from build123d import *

# Parameters (mm, degrees)
SKETCH_1_W          = 160
SKETCH_1_H          = 140
EXTRUDE_1_DEPTH     = 45
SKETCH_2_W          = 160
SKETCH_2_H          = 100
EXTRUDE_2_DEPTH     = 45
SKETCH_3_R          = 12.5
CUT_EXTRUDE_1_DEPTH = 116.433963806
SKETCH_4_R          = 32.5
CUT_EXTRUDE_2_DEPTH = 157.524758425
SKETCH_5_R          = 50
CUT_EXTRUDE_3_DEPTH = 7.5
SKETCH_7_W          = 136
SKETCH_7_H          = 76
CUT_EXTRUDE_4_DEPTH = 25


with BuildPart() as part:
    # Эскиз1 → Бобышка-Вытянуть1 (new body)
    with BuildSketch(Plane.XY):
        Rectangle(SKETCH_1_W, SKETCH_1_H)
    extrude(amount=EXTRUDE_1_DEPTH)

    # Эскиз2 → Бобышка-Вытянуть2 (add)
    with BuildSketch(Plane.XY.offset(45)):
        with Locations((0, 20)):
            Rectangle(SKETCH_2_W, SKETCH_2_H)
    extrude(amount=EXTRUDE_2_DEPTH)

    # Эскиз3 → Вырез-Вытянуть1 (cut, through all)
    with BuildSketch(Plane.XY.offset(45)):
        with Locations((0, -50)):
            Circle(SKETCH_3_R)
    extrude(amount=-CUT_EXTRUDE_1_DEPTH, mode=Mode.SUBTRACT)

    # Эскиз4 → Вырез-Вытянуть2 (cut, through all)
    with BuildSketch(Plane.XZ.offset(30)):
        with Locations((0, 90)):
            Circle(SKETCH_4_R)
    extrude(amount=-CUT_EXTRUDE_2_DEPTH, mode=Mode.SUBTRACT)

    # Эскиз5 → Вырез-Вытянуть3 (cut, symmetric)
    with BuildSketch(Plane(origin=(0, 20, 0), x_dir=(-1, 0, 0), z_dir=(0, -1, 0))):
        with Locations((0, -90)):
            Circle(SKETCH_5_R)
    extrude(amount=CUT_EXTRUDE_3_DEPTH, both=True, mode=Mode.SUBTRACT)

    # Эскиз7 → Вырез-Вытянуть4 (cut)
    with BuildSketch(Plane.XY.offset(90)):
        with Locations((0, 20)):
            Rectangle(SKETCH_7_W, SKETCH_7_H)
    extrude(amount=-CUT_EXTRUDE_4_DEPTH, mode=Mode.SUBTRACT)


solid = part.part
The model under review builds one solid part; all positions refer to its coordinate system, in mm. A direction names the side the tool comes from. Round coordinates to 2 decimals unless told otherwise and drop trailing zeros. Write each loop counter-clockwise with the first axis right and the second up, starting at its lowest first coordinate (ties: lowest second). Pieces come first, ordered by that corner, then holes. Notation, with made-up numbers: (-7.75, 1) - (43.25, 1) arc R27 cw to (43.25, 34) - close; hole circle Ø11 at (64, 35). An arc over 180 degrees is marked (long way). One line per item, written item: value. Start each with the question number.
1. Machinability: for faces 1 (the face through (-0.715, -13.77, 57.508)), 2 (the face through (-0.733, 19.895, 40.005)), 3 (the face through (-1, -63, 45)), which of the approach directions +Z, -Z, +X, -X, +Y, -Y give a long, thin tool a straight path to every point of the face, cutting with its end or side? Answer none if there is none.
2. To check wall thickness, follow L1, parallel to Y at x = 0, z = 11.5; L2, parallel to X at y = 49.5, z = 68; L3, parallel to X at y = 6, z = 60. State the ranges of each line that lie inside material, in increasing order. Write a range as from..to.
3. Clearance check with flat-ended pins moving along their axes: P1, Ø20, axis at x = -1.5, z = 58.5, coming from the -Y side; P2, Ø15, axis at x = 0, y = -50, coming from the -Z side; P3, Ø2, axis at x = 9.5, y = 44.5, coming from the +Z side; P4, Ø4, axis at x = 24.5, y = -1, coming from the +Z side. State where each tip first meets the part, or that it passes through.
4. Consider section A-A on y = -50. Write out the cut boundary in (x, z), and give its area (4 significant figures).
5. The part is to be moulded in two halves that separate along Y. For faces 4 (the face through (-72, 21, 90)), 5 (the face through (-2.71, -62.203, 22.815)), 6 (the face through (-1, -30, 57)), say which applies: released by +Y, released by -Y, zero draft, split by the parting line, or undercut.
6. Consider section D-D on x = 60. Write out the cut boundary in (y, z), and give its area (3 significant figures).
7. Consider section C-C on z = 26.5. Write out the cut boundary in (x, y).
8. Consider section B-B on x = 0. Write out the cut boundary in (y, z), and give its area (3 significant figures).
Checks:
1. face 1: +Z, +Y, -Y
1. face 2: +Z
1. face 3: +Z, +X, -X, -Y
2. L1: y = -70..-62.5, -37.5..70
2. L2: x = -80..-68, 68..80
2. L3: x = -80..-12.5, 12.5..80
3. P1: stops at y = -30
3. P2: passes through
3. P3: stops at z = 59.24
3. P4: stops at z = 65
4. outline: (-80, 0) - (-12.5, 0) - (-12.5, 45) - (-80, 45) - close; (12.5, 0) - (80, 0) - (80, 45) - (12.5, 45) - close
4. area: 6,075 mm^2
5. face 4: zero draft
5. face 5: undercut
5. face 6: released by -Y
6. outline: (-70, 0) - (70, 0) - (70, 90) - (58, 90) - (58, 65) - (-18, 65) - (-18, 90) - (-30, 90) - (-30, 45) - (-70, 45) - close
6. area: 8,900 mm^2
7. outline: (-80, -70) - (80, -70) - (80, 70) - (-80, 70) - close; hole circle Ø25 at (0, -50)
8. outline: (-70, 0) - (-62.5, 0) - (-62.5, 45) - (-70, 45) - close; (-37.5, 0) - (70, 0) - (70, 57.5) - (27.5, 57.5) - (27.5, 40) - (12.5, 40) - (12.5, 57.5) - (-30, 57.5) - (-30, 45) - (-37.5, 45) - close
8. area: 6,160 mm^2
